Check sheet for the modelled part. Datum: model origin and axes. Units: mm. Face numbers are marked on the shaded views. A direction names the side the tool comes from. Coordinates: 2 decimals unless noted, no trailing zeros. Loops run counter-clockwise (first coordinate to the right, second up) from the corner with the lowest first, then second, coordinate; pieces in that order, holes last. Notation, with made-up numbers: (-29.75, 81.25) - (22.25, 81.25) arc R15 ccw to (22.25, 102.25) - close; hole circle Ø10 at (42, 23). An arc over 180 degrees is marked (long way). Answer as a JSON object with one key per item and string values. Group by question number.
from build123d import *

# Parameters (mm, degrees)
SKETCH1_W           = 33
SKETCH1_H           = 36
SKETCH1_R           = 1.6
BOSS_EXTRUDE1_DEPTH = 1.68
SKETCH2_W           = 17.413087774
SKETCH2_H           = 22.744623076
BOSS_EXTRUDE2_DEPTH = 14
SKETCH3_W           = 6
SKETCH3_H           = 6
BOSS_EXTRUDE3_DEPTH = 6.5
SKETCH4_W           = 4.108706104
SKETCH4_H           = 18.978309146
BOSS_EXTRUDE4_DEPTH = 18
SKETCH5_R           = 3.495385022
BOSS_EXTRUDE5_DEPTH = 8
FILLET1_R           = 0.5


with BuildPart() as part:
    # Sketch1 → Boss-Extrude1 (new body)
    with BuildSketch(Plane(origin=(0, 0, 0), x_dir=(1, 0, 0), z_dir=(0, 1, 0))):
        Rectangle(SKETCH1_W, SKETCH1_H)
        with Locations(Location((-13.65, 15.15, 0), (0, 0, 270))):
            Circle(SKETCH1_R, mode=Mode.SUBTRACT)
        with Locations(Location((13.65, 15.15, 0), (0, 0, 270))):
            Circle(SKETCH1_R, mode=Mode.SUBTRACT)
        with Locations(Location((13.65, -15.15, 0), (0, 0, 270))):
            Circle(SKETCH1_R, mode=Mode.SUBTRACT)
        with Locations(Location((-13.65, -15.15, 0), (0, 0, 270))):
            Circle(SKETCH1_R, mode=Mode.SUBTRACT)
    extrude(amount=BOSS_EXTRUDE1_DEPTH)

    # Sketch2 → Boss-Extrude2 (add)
    with BuildSketch(Plane(origin=(0, 1.68, 0), x_dir=(1, 0, 0), z_dir=(0, 1, 0))):
        with Locations((0.354620467, 4.610066075)):
            Rectangle(SKETCH2_W, SKETCH2_H)
    extrude(amount=BOSS_EXTRUDE2_DEPTH)

    # Sketch3 → Boss-Extrude3 (add)
    with BuildSketch(Plane(origin=(0, 15.68, 0), x_dir=(1, 0, 0), z_dir=(0, 1, 0))):
        with Locations((0, 10.308450136)):
            Rectangle(SKETCH3_W, SKETCH3_H)
    extrude(amount=BOSS_EXTRUDE3_DEPTH)

    # Sketch4 → Boss-Extrude4 (add)
    with BuildSketch(Plane(origin=(0, 1.68, 0), x_dir=(1, 0, 0), z_dir=(0, 1, 0))):
        with Locations((-13.096500706, -0.452446803)):
            Rectangle(SKETCH4_W, SKETCH4_H)
    boss_extrude4 = extrude(amount=BOSS_EXTRUDE4_DEPTH)

    # Mirror1: Boss-Extrude4 across plane
    add(boss_extrude4.mirror(Plane(origin=(0, 0, 0), x_dir=(0, 0, 1), z_dir=(1, 0, 0))))

    # Sketch5 → Boss-Extrude5 (add)
    with BuildSketch(Plane(origin=(0, 1.68, 0), x_dir=(1, 0, 0), z_dir=(0, 1, 0))):
        with Locations(Location((7.61678506, -13.414271653, 0), (0, 0, 90))):
            Circle(SKETCH5_R)
        with Locations(Location((0.380282147, -13.414271653, 0), (0, 0, 90))):
            Circle(SKETCH5_R)
    extrude(amount=BOSS_EXTRUDE5_DEPTH)

    # Fillet1
    fillet1_edges = [part.edges().sort_by_distance(p)[0] for p in [
        (7.61678506, 9.68, 16.909656675),
        (0.380282147, 9.68, 16.909656675),
    ]]
    fillet(fillet1_edges, radius=FILLET1_R)


solid = part.part
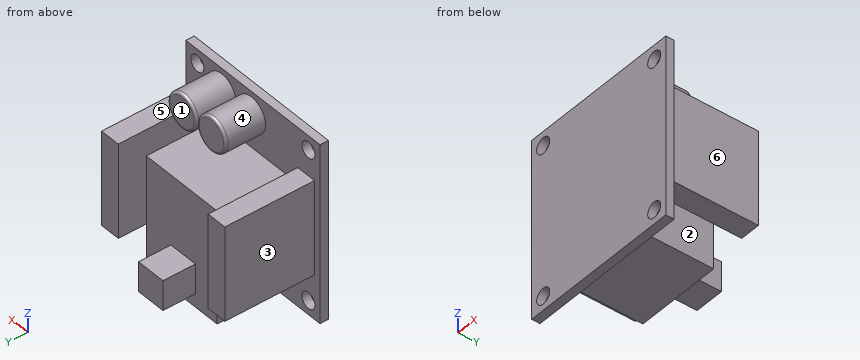
1. Sectioned sample at D-D on y = 11.5. Record the cut outline in (x, z).
2. Sectioned sample at A-A on y = 17.75. Record the cut outline in (x, z), plus the area to 3 significant figures.
3. Release check for a two-part mould opening along X. For the marked faces 4, 5 and 6 record: released by +X, released by -X, zero draft, split by the parting line, or undercut.
4. Sectioned sample at B-B on z = -15.15. Record the cut outline in (x, y), plus the area to 3 significant figures.
5. Material ranges on line 1 (X direction, y = 0.9, z = -15.15); line 2 (X direction, y = 2.75, z = -8); line 3 (X direction, y = 6.5, z = 7), recorded low to high.
6. Sectioned sample at C-C on x = -13.65. Record the cut outline in (y, z).
7. Access from +Z, -Z, +X, -X, +Y, -Y to the whole of each face (thin tool, end or side, straight path). Record for the marked faces 1, 2 and 3.
8. Gauge pin test, flat ends, axial feed: pin 1 (2.5 mm diameter, centred on x = 13.65, z = -15.15, fed in from -Y); pin 2 (3 mm diameter, centred on y = 12.5, z = 5.5, fed in from -X); pin 3 (3 mm diameter, centred on x = 1.5, z = 13, fed in from +Y); pin 4 (5 mm diameter, centred on x = 1, y = 18, fed in from -Z). Record the tip position at first contact, or that the pin passes through.
Answers follow:
{
 "1": {"outline": "(-15.15, -9.04) - (-11.04, -9.04) - (-11.04, 9.94) - (-15.15, 9.94) - close; (-8.35, -15.98) - (9.06, -15.98) - (9.06, 6.76) - (-8.35, 6.76) - close; (11.04, -9.04) - (15.15, -9.04) - (15.15, 9.94) - (11.04, 9.94) - close"},
 "2": {"outline": "(-15.15, -9.04) - (-11.04, -9.04) - (-11.04, 9.94) - (-15.15, 9.94) - close; (-3, -13.31) - (3, -13.31) - (3, -7.31) - (-3, -7.31) - close; (11.04, -9.04) - (15.15, -9.04) - (15.15, 9.94) - (11.04, 9.94) - close", "area": "192 mm^2"},
 "3": {"face 4": "undercut", "face 5": "zero draft", "face 6": "released by +X"},
 "4": {"outline": "(-16.5, 0) - (-15.25, 0) - (-15.25, 1.68) - (-16.5, 1.68) - close; (-12.05, 0) - (12.05, 0) - (12.05, 1.68) - (9.06, 1.68) - (9.06, 15.68) - (-8.35, 15.68) - (-8.35, 1.68) - (-12.05, 1.68) - close; (15.25, 0) - (16.5, 0) - (16.5, 1.68) - (15.25, 1.68) - close", "area": "288 mm^2"},
 "5": {"line 1": "x = -16.5 to -15.25, -12.05 to 12.05, 15.25 to 16.5", "line 2": "x = -15.15 to -11.04, -8.35 to 9.06, 11.04 to 15.15", "line 3": "x = -15.15 to -11.04, 11.04 to 15.15"},
 "6": {"outline": "(0, -18) - (1.68, -18) - (1.68, -16.75) - (0, -16.75) - close; (0, -13.55) - (1.68, -13.55) - (1.68, -9.04) - (19.68, -9.04) - (19.68, 9.94) - (1.68, 9.94) - (1.68, 13.55) - (0, 13.55) - close; (0, 16.75) - (1.68, 16.75) - (1.68, 18) - (0, 18) - close"},
 "7": {"face 1": "+Z, +X, -X, +Y", "face 2": "-Z, +Y", "face 3": "+Z, -Z, -X, +Y"},
 "8": {"pin 1": "passes through", "pin 2": "stops at x = -15.15", "pin 3": "stops at y = 9.68", "pin 4": "stops at z = -15.98"}
}
